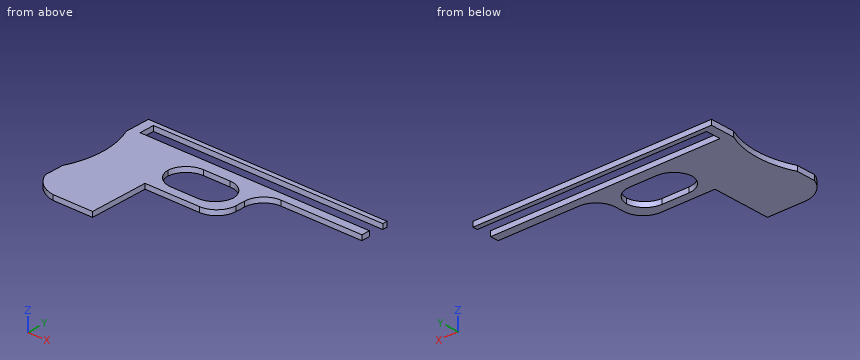
from build123d import *

# Parameters (mm, degrees)
F0_W         = 142.9656147957
F0_H         = 80.8112323284
F1_DEPTH     = 3
F2_W         = 137.4550536275
F2_H         = 8.9848991483
F2_W_2       = 60.0944850594
F2_H_2       = 18.4983238578
F3_DEPTH     = 52.3
F4_W         = 39.2408655025
F4_H         = 21.6958951205
F5_DEPTH     = 25
F6_W         = 3.3521875739
F6_H         = 44.7733802721
F6_W_2       = 40.9712046385
F7_DEPTH     = 25
F8_W         = 102.604271844
F8_H         = 18.422623165
F9_DEPTH     = 25
F10_T1_DEPTH = 3
F10_T3_DEPTH = 60.941125497
F12_DEPTH    = 25
F14_DEPTH    = 25
F16_DEPTH    = 25


# Not quite as in the source:
# - a fillet or chamfer that OpenCascade refuses, or shapes differently, is made with other operations: its cross-section is extruded or revolved along the edge and cut away or added


with BuildPart() as f1:
    # F0 (on Top) → F1 (new body)
    with BuildSketch(Plane.XY):
        Rectangle(F0_W, F0_H)
    extrude(amount=F1_DEPTH)

    # F2 (on face) → F3 (cut)
    with BuildSketch(Plane.XY.offset(3)):
        with Locations((2.7552805841, 33.0591509119)):
            Rectangle(F2_W, F2_H)
        with Locations((41.4355648682, 14.2965670675)):
            Rectangle(F2_W_2, F2_H_2)
    extrude(amount=-F3_DEPTH, mode=Mode.SUBTRACT)

    # F4 (on face) → F5 (cut)
    with BuildSketch(Plane.XY.offset(3)):
        with Locations((-13.8379565906, 10.8479475603)):
            Rectangle(F4_W, F4_H)
    extrude(amount=-F5_DEPTH, mode=Mode.SUBTRACT)

    # F6 (on face) → F7 (cut)
    with BuildSketch(Plane.XY.offset(3)):
        Polygon((98.6725464463, 0), (13.7504395097, 0), (13.7504395097, -5.2010240033), (17.1026270837, -5.2010240033), (17.1026270837, -49.9744042754), (13.7504395097, -49.9744042754), (13.7504395097, -55.2418604493), (98.6725464463, -55.2418604493), align=None)
        with Locations((15.4265332967, -27.5877141394)):
            Rectangle(F6_W, F6_H)
        with Locations((-6.7351628095, -27.5877141394)):
            Rectangle(F6_W_2, F6_H)
    extrude(amount=-F7_DEPTH, mode=Mode.SUBTRACT)

    # F8 (on face) → F9 (cut)
    with BuildSketch(Plane.XY.offset(3)):
        with Locations((62.6904582605, -4.1639064439)):
            Rectangle(F8_W, F8_H)
    extrude(amount=-F9_DEPTH, mode=Mode.SUBTRACT)

    # F10: fillet of radius 11.5882250994 on 7 edges, made by hand

    # F10_s2 → F10_t1 (join)
    with BuildSketch(Plane.XY):
        with BuildLine():
            ThreePointArc((22.9765474379, 23.5457289964), (14.7824348882, 20.1516164467), (11.3883223385, 11.957503897))
            Line((11.3883223385, 11.957503897), (11.3883223385, 23.5457289964))
            Line((11.3883223385, 23.5457289964), (22.9765474379, 23.5457289964))
        make_face()
        with BuildLine():
            ThreePointArc((-15.6325400293, -5.2010240033), (-23.826652579, -8.595136553), (-27.2207651287, -16.7892491027))
            Line((-27.2207651287, -16.7892491027), (-27.2207651287, -5.2010240033))
            Line((-27.2207651287, -5.2010240033), (-15.6325400293, -5.2010240033))
        make_face()
        with BuildLine():
            ThreePointArc((-33.4583893418, 10.1076700211), (-30.0642767921, 18.3017825708), (-21.8701642424, 21.6958951205))
            Line((-21.8701642424, 21.6958951205), (-33.4583893418, 21.6958951205))
            Line((-33.4583893418, 21.6958951205), (-33.4583893418, 10.1076700211))
        make_face()
        with BuildLine():
            ThreePointArc((-5.8057489387, 0), (2.388363611, 3.3941125497), (5.7824761607, 11.5882250994))
            Line((5.7824761607, 11.5882250994), (5.7824761607, 0))
            Line((5.7824761607, 0), (-5.8057489387, 0))
        make_face()
        with BuildLine():
            ThreePointArc((-33.4583893418, 11.5882250994), (-30.0642767921, 3.3941125497), (-21.8701642424, 0))
            Line((-21.8701642424, 0), (-33.4583893418, 0))
            Line((-33.4583893418, 0), (-33.4583893418, 11.5882250994))
        make_face()
        with BuildLine():
            ThreePointArc((5.7824761607, 10.1076700211), (2.388363611, 18.3017825708), (-5.8057489387, 21.6958951205))
            Line((-5.8057489387, 21.6958951205), (5.7824761607, 21.6958951205))
            Line((5.7824761607, 21.6958951205), (5.7824761607, 10.1076700211))
        make_face()
    extrude(amount=F10_T1_DEPTH)

    # F10_s4 → F10_t3 (cut)
    with BuildSketch(Plane.XY.offset(-28.9705627485)):
        with BuildLine():
            ThreePointArc((-0.1999027609, -5.2010240033), (7.9942097888, -1.8069114536), (11.3883223385, 6.3872010961))
            Line((11.3883223385, 6.3872010961), (11.3883223385, -5.2010240033))
            Line((11.3883223385, -5.2010240033), (-0.1999027609, -5.2010240033))
        make_face()
    extrude(amount=F10_T3_DEPTH, mode=Mode.SUBTRACT)

    # F11 (on face) → F12 (cut)
    with BuildSketch(Plane.XY.offset(3)):
        with BuildLine():
            Line((-71.4828073978, 25.5012605339), (-71.4828073978, -17.3091441393))
            ThreePointArc((-71.4828073978, -17.3091441393), (-66.7668008007, 4.0960581973), (-71.4828073978, 25.5012605339))
        make_face()
    extrude(amount=-F12_DEPTH, mode=Mode.SUBTRACT)

    # F13 (on face) → F14 (cut)
    with BuildSketch(Plane.XY.offset(3)):
        with BuildLine():
            ThreePointArc((-21.3245461018, -6.6952891353), (-30.1185964093, -13.4662376926), (-27.2207651287, -24.1799503565))
            Line((-27.2207651287, -24.1799503565), (-27.2207651287, -16.7892491027))
            ThreePointArc((-27.2207651287, -16.7892491027), (-25.6387183355, -10.944306275), (-21.3245461018, -6.6952891353))
        make_face()
        with BuildLine():
            ThreePointArc((-27.2207651287, -32.8327932205), (-29.4171017882, -37.101902666), (-32.9005867243, -40.4056161642))
            Line((-32.9005867243, -40.4056161642), (-27.2207651287, -40.4056161642))
            Line((-27.2207651287, -40.4056161642), (-27.2207651287, -32.8327932205))
        make_face()
        with BuildLine():
            ThreePointArc((-56.574376872, -40.4056161642), (-65.5880780241, -36.6447482344), (-71.4828073978, -28.8573801517))
            Line((-71.4828073978, -28.8573801517), (-71.4828073978, -40.4056161642))
            Line((-71.4828073978, -40.4056161642), (-56.574376872, -40.4056161642))
        make_face()
    extrude(amount=-F14_DEPTH, mode=Mode.SUBTRACT)

    # F15 (on face) → F16 (cut)
    with BuildSketch(Plane.XY.offset(3)):
        with BuildLine():
            Line((-32.9005867243, -5.2010240033), (-32.9005867243, -40.4056161642))
            ThreePointArc((-32.9005867243, -40.4056161642), (-29.4171017882, -37.101902666), (-27.2207651287, -32.8327932205))
            Line((-27.2207651287, -32.8327932205), (-27.2207651287, -24.1799503565))
            ThreePointArc((-27.2207651287, -24.1799503565), (-30.1185964093, -13.4662376926), (-21.3245461018, -6.6952891353))
            ThreePointArc((-21.3245461018, -6.6952891353), (-18.5749778542, -5.5808138595), (-15.6325400293, -5.2010240033))
            Line((-15.6325400293, -5.2010240033), (-32.9005867243, -5.2010240033))
        make_face()
    extrude(amount=-F16_DEPTH, mode=Mode.SUBTRACT)


solid = f1.part
The model under review builds one solid part; all positions refer to its coordinate system, in mm. Round coordinates to 2 decimals unless told otherwise and drop trailing zeros. Loops run counter-clockwise (first coordinate to the right, second up) from the corner with the lowest first, then second, coordinate; pieces in that order, holes last. Notation, with made-up numbers: M 63.5,-35.75 L 97.5,-35.75 A32 ccw 97.5,-3.75 Z; hole C 73.5,25 d4. An arc over 180 degrees is marked long. Answer as CSV lines item,"result". Start each with the question number.
Item 1: Consider section A-A (x = 43). Write out the cut boundary in (y, z), then the cut area to 3 significant figures.
Item 2: Consider section C-C (y = 4). Write out the cut boundary in (x, z).
Item 3: Wall thickness on line 1 (Y direction, x = -22, z = 1.8); line 2 (Y direction, x = 35, z = 1.1); line 3 (Y direction, x = -4, z = 1): over which ranges is each line inside the solid? List them lowest first. Write a range as [from, to].
Item 4: Consider section D-D (x = -23.5). Write out the cut boundary in (y, z).
Item 5: Consider section B-B (z = 0.5). Write out the cut boundary in (x, y).
Item 6: Insertion check: P1, Ø1.5, axis at y = 10, z = 1, coming from the +X side; P2, Ø1.5, axis at y = 33, z = 1.5, coming from the +X side; P3, Ø1.5, axis at x = 40, z = 1.5, coming from the -Y side. Each pin has a flat end and moves straight along its axis. Give the tip position at first contact, or say it passes through.
Answer:
1,outline,"M 23.55,0 L 28.57,0 L 28.57,3 L 23.55,3 Z; M 37.55,0 L 40.41,0 L 40.41,3 L 37.55,3 Z"
1,area,"23.6 mm^2"
2,outline,"M -66.77,0 L -30.63,0 L -30.63,3 L -66.77,3 Z; M 2.95,0 L 11.14,0 L 11.14,3 L 2.95,3 Z"
3,line 1,"y = [-5.2, 0], [21.7, 28.57], [37.55, 40.41]"
3,line 2,"y = [23.55, 28.57], [37.55, 40.41]"
3,line 3,"y = [-5.2, 0.14], [21.55, 28.57], [37.55, 40.41]"
4,outline,"M -5.2,0 L 0.12,0 L 0.12,3 L -5.2,3 Z; M 21.58,0 L 28.57,0 L 28.57,3 L 21.58,3 Z; M 37.55,0 L 40.41,0 L 40.41,3 L 37.55,3 Z"
5,outline,"M -71.48,-28.86 A18.73 ccw -56.57,-40.41 L -32.9,-40.41 L -32.9,-5.2 L -0.2,-5.2 A11.59 ccw 11.39,6.39 L 11.39,11.96 A11.59 cw 22.98,23.55 L 71.48,23.55 L 71.48,28.57 L -65.97,28.57 L -65.97,37.55 L 71.48,37.55 L 71.48,40.41 L -71.48,40.41 L -71.48,25.5 A50.94 cw -71.48,-17.31 Z; hole M -33.43,10.85 A11.59 ccw -21.87,0 L -5.81,0 A11.59 ccw 5.76,10.85 A11.59 ccw -5.81,21.7 L -21.87,21.7 A11.59 ccw Z"
6,P1,"stops at x = 11.39"
6,P2,"stops at x = -65.97"
6,P3,"stops at y = 23.55"
